Could you check a few things on this model? Use its own coordinates, in mm. Face numbers are marked on the shaded views. A direction names the side the tool comes from. Coordinates: 2 decimals unless noted, no trailing zeros. Write each loop counter-clockwise with the first axis right and the second up, starting at its lowest first coordinate (ties: lowest second). Pieces come first, ordered by that corner, then holes.
```python
from build123d import *

# Parameters (mm, degrees)
SKETCH_1_W          = 10
SKETCH_1_H          = 19.9
EXTRUDE_1_DEPTH     = 29.9
SKETCH_4_R          = 6
EXTRUDE_2_DEPTH     = 33
SKETCH_7_R          = 2
CUT_EXTRUDE_1_DEPTH = 9.6


with BuildPart() as part:
    # Эскиз1 → Бобышка-Вытянуть1 (new body)
    with BuildSketch(Plane(origin=(0, 0, 0), x_dir=(1, 0, 0), z_dir=(0, 1, 0))):
        Rectangle(SKETCH_1_W, SKETCH_1_H)
    extrude(amount=EXTRUDE_1_DEPTH)

    # Эскиз4 → Бобышка-Вытянуть2 (add)
    with BuildSketch(Plane(origin=(5, 0, 0), x_dir=(0, 0, -1), z_dir=(1, 0, 0))):
        with Locations((0, 14.95)):
            Circle(SKETCH_4_R)
    extrude(amount=EXTRUDE_2_DEPTH)

    # Эскиз7 → Вырез-Вытянуть1 (cut)
    with BuildSketch(Plane.ZY.offset(5)):
        with Locations((0, 14.95)):
            Circle(SKETCH_7_R)
    extrude(amount=-CUT_EXTRUDE_1_DEPTH, mode=Mode.SUBTRACT)


solid = part.part
```
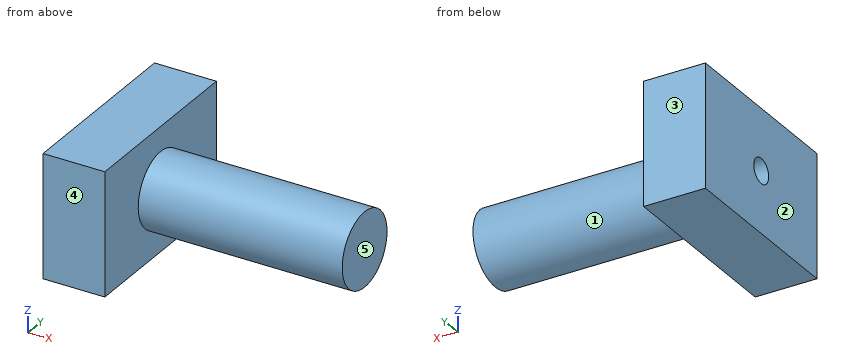
Item 1: Which directions (+Z, -Z, +X, -X, +Y, -Y) give clear straight access to the entire face, cutting with the end or side of a thin tool? Please do the marked faces 1 and 2.
Item 2: I want a section at C-C, the plane y = 14.95. List the corners of the cut face in (x, z) for me, then the cut area to 3 significant figures.
Item 3: I want a section at D-D, the plane x = 33.5. List the corners of the cut face in (y, z) for me, then the cut area to 3 significant figures.
Item 4: If we mould it in two halves opening along Y, with no side actions, what happens to the marked faces 3, 4 and 5? For each: released by +Y, released by -Y, zero draft, split by the parting line, or undercut.
Item 5: If I drill on line 1 along Y through (x, z) = (1.5, 0); line 2 along X through (y, z) = (5.75, -3.5); line 3 along Y through (x, z) = (28.5, 4.75), over which ranges is the centre line in solid material (lowest first)?
Item 6: I want a section at B-B, the plane x = -0.5. List the corners of the cut face in (y, z) for me.
Item 7: I want a section at A-A, the plane z = 0. List the corners of the cut face in (x, y) for me.
Item 8: Will these pins go through, and if not, where does the flat tip stop? pin 1 Ø4 at (x, y) = (21, 14.5) entering from -Z; pin 2 Ø3 at (y, z) = (14.5, 0) entering from -X; pin 3 Ø1 at (y, z) = (8.5, -3.5) entering from +X.
Taken from the geometry:
1. face 1: +X
1. face 2: +Z, -Z, -X, +Y, -Y
2. outline: (-5, -9.95) - (5, -9.95) - (5, -6) - (38, -6) - (38, 6) - (5, 6) - (5, 9.95) - (-5, 9.95) - (-5, 2) - (4.6, 2) - (4.6, -2) - (-5, -2) - close
2. area: 557 mm2
3. outline: circle Ø12 at (14.95, 0)
3. area: 113 mm2
4. face 3: released by +Y
4. face 4: released by -Y
4. face 5: zero draft
5. line 1: y = 0 to 12.95, 16.95 to 29.9
5. line 2: x = -5 to 5
5. line 3: y = 11.28 to 18.62
6. outline: (0, -9.95) - (29.9, -9.95) - (29.9, 9.95) - (0, 9.95) - close; hole circle Ø4 at (14.95, 0)
7. outline: (-5, 0) - (5, 0) - (5, 8.95) - (38, 8.95) - (38, 20.95) - (5, 20.95) - (5, 29.9) - (-5, 29.9) - (-5, 16.95) - (4.6, 16.95) - (4.6, 12.95) - (-5, 12.95) - close
8. pin 1: stops at z = -6
8. pin 2: stops at x = 4.6
8. pin 3: stops at x = 5
